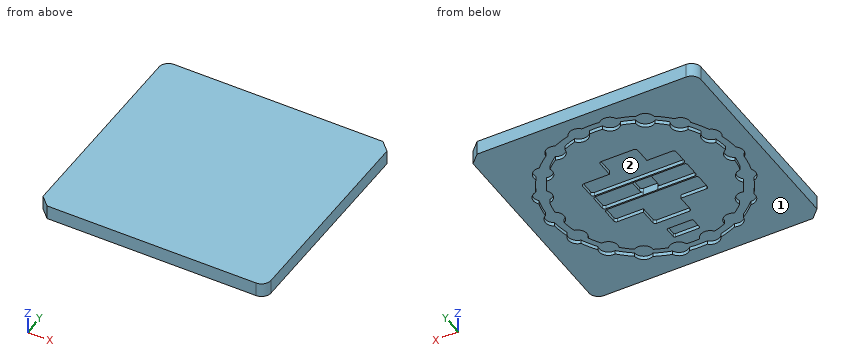
```python
from build123d import *

# Parameters (mm, degrees)
F2_DEPTH  = 19.05
F3_SIZE   = 12.7
F1_W      = 50
F1_H      = 0.2995532098
F1_H_2    = 0.7460711968
F4_DEPTH  = 5
F5_R      = 12.5
F6_DEPTH  = 5
F7_R      = 127
F7_R_2    = 114.3
F8_DEPTH  = 5
F10_DEPTH = 5
F12_DEPTH = 10


with BuildPart() as f2:
    # F0 (on Top) → F2 (new body)
    with BuildSketch(Plane.XY):
        with BuildLine():
            Line((-152.4, -147.4406201886), (139.7, -147.4406201886))
            ThreePointArc((139.7, -147.4406201886), (148.6802561211, -143.7208763097), (152.4, -134.7406201886))
            Line((152.4, -134.7406201886), (152.4, 147.4406201886))
            Line((152.4, 147.4406201886), (-139.7, 147.4406201886))
            ThreePointArc((-139.7, 147.4406201886), (-148.6802561211, 143.7208763097), (-152.4, 134.7406201886))
            Line((-152.4, 134.7406201886), (-152.4, -147.4406201886))
        make_face()
    extrude(amount=F2_DEPTH)

    # F3
    f3_edges = [f2.edges().sort_by_distance(p)[0] for p in [
        (-152.4, -147.44062, 9.525),
        (152.4, 147.44062, 9.525),
    ]]
    chamfer(f3_edges, length=F3_SIZE)

    # F1 (on Top) → F4 (cut)
    with BuildSketch(Plane.XY):
        with BuildLine():
            Line((-59.325, -12.5), (59.325, -12.5))
            ThreePointArc((59.325, -12.5), (61.5700640303, -11.5700640303), (62.5, -9.325))
            Line((62.5, -9.325), (62.5, 9.325))
            ThreePointArc((62.5, 9.325), (61.5700640303, 11.5700640303), (59.325, 12.5))
            Line((59.325, 12.5), (-59.325, 12.5))
            ThreePointArc((-59.325, 12.5), (-61.5700640303, 11.5700640303), (-62.5, 9.325))
            Line((-62.5, 9.325), (-62.5, -9.325))
            ThreePointArc((-62.5, -9.325), (-61.5700640303, -11.5700640303), (-59.325, -12.5))
        make_face()
        with BuildLine():
            Line((-59.325, 14.37484), (59.325, 14.37484))
            ThreePointArc((59.325, 14.37484), (61.5700640303, 15.3047759697), (62.5, 17.54984))
            Line((62.5, 17.54984), (62.5, 36.19984))
            ThreePointArc((62.5, 36.19984), (61.5700640303, 38.4449040303), (59.325, 39.37484))
            Line((59.325, 39.37484), (24.8259999848, 39.37484))
            Line((24.8259999848, 39.37484), (24.8259999848, 39.0752867902))
            Line((24.8259999848, 39.0752867902), (-25.1740000152, 39.0752867902))
            Line((-25.1740000152, 39.0752867902), (-25.1740000152, 39.37484))
            Line((-25.1740000152, 39.37484), (-59.325, 39.37484))
            ThreePointArc((-59.325, 39.37484), (-61.5700640303, 38.4449040303), (-62.5, 36.19984))
            Line((-62.5, 36.19984), (-62.5, 17.54984))
            ThreePointArc((-62.5, 17.54984), (-61.5700640303, 15.3047759697), (-59.325, 14.37484))
        make_face()
        with Locations((-0.1740000152, 39.2250633951)):
            Rectangle(F1_W, F1_H)
        with BuildLine():
            Line((-25.1740000152, 39.37484), (24.8259999848, 39.37484))
            Line((24.8259999848, 39.37484), (24.8259999848, 60.9002867902))
            ThreePointArc((24.8259999848, 60.9002867902), (23.896064015, 63.1453508205), (21.6509999848, 64.0752867902))
            Line((21.6509999848, 64.0752867902), (-21.9990000152, 64.0752867902))
            ThreePointArc((-21.9990000152, 64.0752867902), (-24.2440640455, 63.1453508205), (-25.1740000152, 60.9002867902))
            Line((-25.1740000152, 60.9002867902), (-25.1740000152, 39.37484))
        make_face()
        with BuildLine():
            ThreePointArc((59.325, -39.37484), (61.5700640303, -38.4449040303), (62.5, -36.19984))
            Line((62.5, -36.19984), (62.5, -17.54984))
            ThreePointArc((62.5, -17.54984), (61.5700640303, -15.3047759697), (59.325, -14.37484))
            Line((59.325, -14.37484), (-59.325, -14.37484))
            ThreePointArc((-59.325, -14.37484), (-61.5700640303, -15.3047759697), (-62.5, -17.54984))
            Line((-62.5, -17.54984), (-62.5, -36.19984))
            ThreePointArc((-62.5, -36.19984), (-61.5700640303, -38.4449040303), (-59.325, -39.37484))
            Line((-59.325, -39.37484), (-25.1740000152, -39.37484))
            Line((-25.1740000152, -39.37484), (-25.1740000152, -38.6287688032))
            Line((-25.1740000152, -38.6287688032), (24.8259999848, -38.6287688032))
            Line((24.8259999848, -38.6287688032), (24.8259999848, -39.37484))
            Line((24.8259999848, -39.37484), (59.325, -39.37484))
        make_face()
        with BuildLine():
            Line((24.8259999848, -61.4887688032), (24.8259999848, -39.37484))
            Line((24.8259999848, -39.37484), (-25.1740000152, -39.37484))
            Line((-25.1740000152, -39.37484), (-25.1740000152, -61.4887688032))
            ThreePointArc((-25.1740000152, -61.4887688032), (-24.2440640455, -63.7338328334), (-21.9990000152, -64.6637688032))
            Line((-21.9990000152, -64.6637688032), (21.6509999848, -64.6637688032))
            ThreePointArc((21.6509999848, -64.6637688032), (23.896064015, -63.7338328334), (24.8259999848, -61.4887688032))
        make_face()
        with Locations((-0.1740000152, -39.0018044016)):
            Rectangle(F1_W, F1_H_2)
    extrude(amount=F4_DEPTH, mode=Mode.SUBTRACT)

    # F5 (on Top) → F6 (cut)
    with BuildSketch(Plane.XY):
        with Locations((-118.9195587855, -0.6876965701)):
            Circle(F5_R)
        with Locations((-111.4739967474, -41.5381840536)):
            Circle(F5_R)
        with Locations((-90.5057674586, -77.3785535018)):
            Circle(F5_R)
        with Locations((-58.5439488294, -103.8859274119)):
            Circle(F5_R)
        with Locations((-19.4436078927, -117.8631252832)):
            Circle(F5_R)
        with Locations((22.079177175, -117.6242907708)):
            Circle(F5_R)
        with Locations((61.0161456833, -103.1982308418)):
            Circle(F5_R)
        with Locations((92.6709245819, -76.3249412296)):
            Circle(F5_R)
        with Locations((113.2254803607, -40.2457372689)):
            Circle(F5_R)
        with Locations((120.2006302398, 0.6876965701)):
            Circle(F5_R)
        with Locations((112.7550682017, 41.5381840536)):
            Circle(F5_R)
        with Locations((91.7868389128, 77.3785535018)):
            Circle(F5_R)
        with Locations((59.8250202836, 103.8859274119)):
            Circle(F5_R)
        with Locations((20.724679347, 117.8631252832)):
            Circle(F5_R)
        with Locations((-20.7981057207, 117.6242907708)):
            Circle(F5_R)
        with Locations((-59.735074229, 103.1982308418)):
            Circle(F5_R)
        with Locations((-91.3898531276, 76.3249412296)):
            Circle(F5_R)
        with Locations((-111.9444089064, 40.2457372689)):
            Circle(F5_R)
    extrude(amount=F6_DEPTH, mode=Mode.SUBTRACT)

    # F7 (on Top) → F8 (cut)
    with BuildSketch(Plane.XY):
        Circle(F7_R)
        Circle(F7_R_2, mode=Mode.SUBTRACT)
    extrude(amount=F8_DEPTH, mode=Mode.SUBTRACT)

    # F9 (on Top) → F10 (cut)
    with BuildSketch(Plane.XY):
        with BuildLine():
            ThreePointArc((-18.1759242915, -95.255201998), (-17.7109563066, -96.3777340131), (-16.5884242915, -96.842701998))
            Line((-16.5884242915, -96.842701998), (15.1615757085, -96.842701998))
            ThreePointArc((15.1615757085, -96.842701998), (16.2841077237, -96.3777340131), (16.7490757085, -95.255201998))
            Line((16.7490757085, -95.255201998), (16.7490757085, -80.967701998))
            ThreePointArc((16.7490757085, -80.967701998), (16.2841077237, -79.8451699828), (15.1615757085, -79.380201998))
            Line((15.1615757085, -79.380201998), (-16.5884242915, -79.380201998))
            ThreePointArc((-16.5884242915, -79.380201998), (-17.7109563066, -79.8451699828), (-18.1759242915, -80.967701998))
            Line((-18.1759242915, -80.967701998), (-18.1759242915, -95.255201998))
        make_face()
    extrude(amount=F10_DEPTH, mode=Mode.SUBTRACT)

    # F11 (on Top) → F12 (cut)
    with BuildSketch(Plane.XY):
        with BuildLine():
            ThreePointArc((12.5, 9.4338746626), (11.5700640303, 11.6789386929), (9.325, 12.6088746626))
            Line((9.325, 12.6088746626), (-9.325, 12.6088746626))
            ThreePointArc((-9.325, 12.6088746626), (-11.5700640303, 11.6789386929), (-12.5, 9.4338746626))
            Line((-12.5, 9.4338746626), (-12.5, -9.4338746626))
            ThreePointArc((-12.5, -9.4338746626), (-11.5700640303, -11.6789386929), (-9.325, -12.6088746626))
            Line((-9.325, -12.6088746626), (9.325, -12.6088746626))
            ThreePointArc((9.325, -12.6088746626), (11.5700640303, -11.6789386929), (12.5, -9.4338746626))
            Line((12.5, -9.4338746626), (12.5, 9.4338746626))
        make_face()
    extrude(amount=F12_DEPTH, mode=Mode.SUBTRACT)


solid = f2.part
```
Verification items for the finished model (mm, model axes). Face numbers are marked on the shaded views. Round coordinates to 2 decimals unless told otherwise and drop trailing zeros. Order: outer loops, then holes, each group sorted by start corner. A loop starts at its lowest first (then second) coordinate and runs counter-clockwise, first axis right, second up. Notation, with made-up numbers: (55, 15) - (91, 15) arc R25 ccw to (91, 35) - close; hole circle Ø7 at (18.25, 51.5). An arc over 180 degrees is marked (long way). Use CSV: the item, a comma, the result in double quotes. Start each with the question number.
1) Mould release check, pull along Y, two halves, no side actions. Record for the marked faces 1 and 2: +Y half, -Y half, draft (parallel to the pull), parting line (faces both ways), or undercut.
2) Thickness scan on L1, parallel to Y at x = -59, z = 3.5; L2, parallel to X at y = -37.5, z = 1.75; L3, parallel to X at y = -59, z = 1.75. Record the ranges inside material, lowest first.
3) Section check A-A, the plane x = 2. Record the cut outline in (y, z), plus the area to 3 significant figures.
4) Go/stop test with flat-tipped pins: P1, Ø20, axis at x = -41.5, y = -3, coming from the -Z side; P2, Ø12, axis at x = -108, y = 41, coming from the -Z side. Record where each tip stops, or that it passes through.
Answers:
1,face 1,"draft"
1,face 2,"undercut"
2,L1,"y = -147.44 to -116.38, -91.39 to -39.37, -14.37 to -12.5, 12.5 to 14.37, 39.37 to 90.72, 115.68 to 147.44"
2,L2,"x = -152.4 to -123.3, -99.64 to -62.22, 62.22 to 101.03, 125.42 to 152.4"
2,L3,"x = -152.4 to -112.46, -97.9 to -25.17, 24.83 to 97.9, 112.46 to 152.4"
3,outline,"(-147.44, 0) - (-126.98, 0) - (-126.98, 5) - (-114.28, 5) - (-114.28, 0) - (-96.84, 0) - (-96.84, 5) - (-79.38, 5) - (-79.38, 0) - (-64.66, 0) - (-64.66, 5) - (-14.37, 5) - (-14.37, 0) - (-12.61, 0) - (-12.61, 10) - (12.61, 10) - (12.61, 0) - (14.37, 0) - (14.37, 5) - (64.08, 5) - (64.08, 0) - (114.28, 0) - (114.28, 5) - (126.98, 5) - (126.98, 0) - (147.44, 0) - (147.44, 19.05) - (-147.44, 19.05) - close"
3,area,"4,650 mm²"
4,P1,"stops at z = 0"
4,P2,"stops at z = 5"
